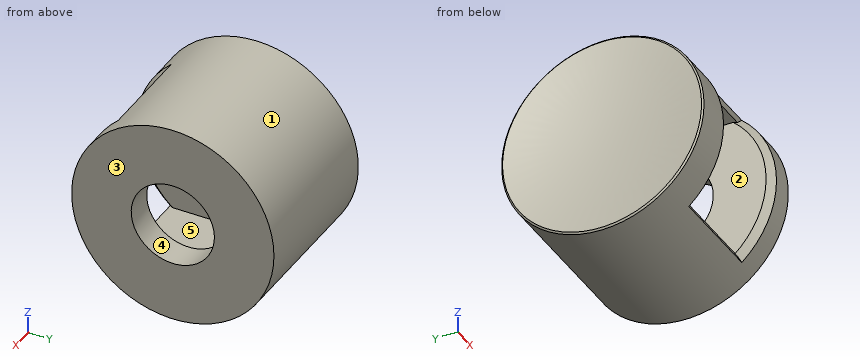
Autodesk Inventor part; units mm, degrees
ref_plane "YZ Plane" through (0, 0, 0) normal (1, 0, 0) x (0, 1, 0)
ref_plane "XZ Plane" through (0, 0, 0) normal (0, 1, 0) x (-1, 0, 0)
ref_plane "XY Plane" through (0, 0, 0) normal (0, 0, 1) x (1, 0, 0)
sketch "Эскиз1" plane through (0, 0, 0) normal (1, 0, 0) x (0, 1, 0)
  circle A0 centre (0, 0) radius 2.067 construction
  circle A1 centre (0, 0) radius 5
  circle A2 centre (0, 0) radius 6
  circle A3 centre (0, 0) radius 2.467
  point P0 (0, 0)
  dimension "d1" = 10
  dimension "d2" = 12
extrude "Выдавливание1" add sketch "Эскиз1" along normal blind 6.7 contours A2
sketch "Эскиз4" plane through (0, 0, 0) normal (-1, 0, 0) x (0, 0, 1)
  circle A0 centre (0, 0) radius 6
  circle A1 centre (0, 0) radius 5
  point P0 (0, 0)
extrude "Выдавливание2" add sketch "Эскиз4" along normal blind 2.64 contours A0 | A1
ref_plane "РабПлоскость1" through (0, 0, 0) normal (0, 1, 0) x (-1, 0, 0)
sketch "Эскиз5" plane through (0, 0, 0) normal (0, 1, 0) x (-1, 0, 0)
  line L0 (2.64, -6) -> (-6.7, -6)
  line L1 (-5, 6) -> (0, 6)
  line L2 (0, 6) -> (0, -6)
  line L3 (0, -6) -> (-5, -6)
  line L4 (-5, -6) -> (-5, 6)
  line L5 (2.64, 6) -> (-6.7, 6)
  line L6 (0, 6) -> (0, -6)
  point P0 (0, 0)
  dimension "d7" = 5
extrude "Выдавливание3" cut sketch "Эскиз5" against normal through all
sketch "Эскиз6" plane through (5, 0, 5) normal (-1, 0, 0) x (0, 0, 1)
  circle A0 centre (-5, 0) radius 5
  circle A1 centre (-5, 0) radius 2.467
extrude "Выдавливание4" add sketch "Эскиз6" against normal up to surface (1.7 mm away)
sketch "Эскиз7" plane through (5, 0, 5) normal (-1, 0, 0) x (0, 0, 1)
  line L0 (-1, 0) -> (-1, -2.3094)
  line L1 (-9, -2.3094) -> (-9, 0)
  circle A0 centre (-5, 0) radius 6
  line L2 (-0.75, -4.2353) -> (-0.75, -2.6339)
  line L3 (1, 0) -> (0, 0)
  line L4 (-10, 0) -> (-11, 0)
  line L5 (-9.25, -2.6339) -> (-9.25, -4.2353)
  line L6 (-0.75, -2.6339) -> (-0.75, 4.2353)
  line L7 (-9.25, -2.6339) -> (-9.25, 4.2353)
  point P0 (-5, 0)
  point P1 (-9.25, -3.4346)
  dimension "d12" = 0.25
  dimension "d13" = 0.25
extrude "Выдавливание5" add sketch "Эскиз7" along normal up to surface (5 mm away) contours A0 L2 L6 | L7 L5 A0
chamfer "Фаска1" distance 0.4 angle 45 4 edges at (5, -6, 0) (2.5, -4.2353, 4.25) (2.5, -4.2353, -4.25) (0, -6, 0)
ref_plane "РабПлоскость2" through (0, 0, 0) normal (-1, 0, 0) x (0, 0, 1)
ref_plane "РабПлоскость3" through (0, 0, 0) normal (0, 1, 0) x (-1, 0, 0)
sketch "Эскиз9" plane through (0, 0, 0) normal (0, 1, 0) x (-1, 0, 0)
  line L0 (2.64, -6) -> (2.64, 6)
  arc A0 (2.64, 6) -> (2.64, -6) centre (47.44, 0) ccw
  line L1 (2.24, 0) -> (2.64, 0)
  point P0 (0, 0)
  dimension "d19" = 0.4
revolve "Вращение1" cut sketch "Эскиз9" angle 360 about axis through (-2.24, 0, 0) along (-1, 0, 0) picked at (2.566, 3.3355) contours L1 A0 L0
chamfer "Фаска2" distance 0.1 angle 45 1 edges at (-2.64, 0, -6)
properties part number "kicker"
CAD build for the part. Positions are in the model's coordinates, mm. Face numbers are marked on the shaded views. A direction names the side the tool comes from. Round coordinates to 2 decimals unless told otherwise and drop trailing zeros. Write each loop counter-clockwise with the first axis right and the second up, starting at its lowest first coordinate (ties: lowest second). Pieces come first, ordered by that corner, then holes. Notation, with made-up numbers: (-8, 6.5) -> (9, 6.5) arc R34 ccw to (9, 45.5) -> close; hole circle Ø1 at (22.5, 86). An arc over 180 degrees is marked (long way). Answer as a JSON object with one key per item and string values.
(1) Probe probe 1 along Y at (x, z) = (5.6, 0); probe 2 along X at (y, z) = (0, -3.5); probe 3 along Z at (x, y) = (2.5, 0.75). List the from-to ranges inside material, lowest first. Write a range as [from, to].
Reported:
{"probe 1": "y = [-6, -2.47], [2.47, 6]", "probe 2": "x = [-2.38, 0], [5, 6.7]", "probe 3": "z = [-5.95, -4.25], [4.25, 5.95]"}
(2) Two-plate mould, pull along X, no slides. Class the marked faces 3, 4 and 5: +X half, -X half, draft (parallel to the pull), parting line (faces both ways), or undercut.
Reported:
{"face 3": "+X half", "face 4": "draft", "face 5": "undercut"}
(3) Which spindle directions (+Z, -Z, +X, -X, +Y, -Y) get a long thin tool onto all of the face, cutting with end or side? Do the marked faces 1 and 2. Say none if no direction does.
Reported:
{"face 1": "+X, -X", "face 2": "-Y"}
(4) Pin check, flat tips, straight feed: P1, Ø4.5, axis at y = -1, z = -2, coming from the -X side; P2, Ø1.5, axis at x = 1, z = -1.5, coming from the +Y side; P3, Ø4, axis at x = 3.5, z = -4, coming from the -Y side. Stop position of each tip, or through.
Reported:
{"P1": "stops at x = -2.46", "P2": "stops at y = 5.95", "P3": "stops at y = -5"}
(5) Band-saw the part on A-A, the plane x = 3. List the corners of the cut face in (y, z).
Reported:
{"outline": "(-3.94, -4.52) arc R6 ccw (long way) to (-3.94, 4.52) -> (-3.84, 4.25) -> (2.63, 4.25) arc R5 cw to (2.63, -4.25) -> (-3.84, -4.25) -> close"}
